Could you check a few things on this model? Use its own coordinates, in mm. Face numbers are marked on the shaded views. A direction names the side the tool comes from. Give positions to 0.01 mm unless a question says otherwise; leave off trailing zeros. Write each loop counter-clockwise with the first axis right and the second up, starting at its lowest first coordinate (ties: lowest second). Pieces come first, ordered by that corner, then holes. Notation, with made-up numbers: (-34.5, 84) - (-15.5, 84) arc R31 ccw to (-15.5, 119) - close; hole circle Ø3 at (35, 14.25). An arc over 180 degrees is marked (long way). Answer as a JSON object with one key per item and string values. Group by question number.
```python
from build123d import *

# Parameters (mm, degrees)
F1_DEPTH = 7.366
F2_T     = -1.27
F4_DEPTH = 0.762


with BuildPart() as f1:
    # F0 (on Top) → F1 (new body)
    with BuildSketch(Plane.XY):
        Polygon((14.39459, 28.100452), (3.467799, 28.100452), (-1.228805, 15.256678), (3.467799, 3.563094), (8.931195, 3.563094), (14.39459, 3.563094), (19.091195, 15.256678), align=None)
    extrude(amount=F1_DEPTH)

    # F2
    f2_openings = [f1.faces().sort_by_distance(p)[0] for p in [
        (8.931195, 28.100452, 3.683),
        (16.742892, 21.678565, 3.683),
        (16.742892, 9.409886, 3.683),
        (1.119497, 21.678565, 3.683),
        (1.119497, 9.409886, 3.683),
    ]]
    offset(amount=F2_T, openings=f2_openings)

    # F3 (on face) → F4 (join)
    with BuildSketch(Plane.XY.offset(7.366)):
        Polygon((3.955232, 13.371391), (13.296179, 13.371391), (8.625706, 21.460889), align=None)
        with BuildLine():
            ThreePointArc((7.451111, 14.032797), (7.055542, 15.560872), (8.146025, 16.702071))
            Line((8.146025, 16.702071), (8.146025, 14.032797))
            Line((8.146025, 14.032797), (7.451111, 14.032797))
        make_face(mode=Mode.SUBTRACT)
        with BuildLine():
            ThreePointArc((9.105387, 16.702071), (10.195869, 15.560872), (9.8003, 14.032797))
            Line((9.8003, 14.032797), (9.105387, 14.032797))
            Line((9.105387, 14.032797), (9.105387, 16.702071))
        make_face(mode=Mode.SUBTRACT)
        with BuildLine():
            Line((6.813301, 14.032797), (5.10082, 14.032797))
            Line((5.10082, 14.032797), (8.146025, 19.307246))
            Line((8.146025, 19.307246), (8.146025, 17.227563))
            ThreePointArc((8.146025, 17.227563), (6.659733, 15.972221), (6.813301, 14.032797))
        make_face(mode=Mode.SUBTRACT)
        with BuildLine():
            Line((9.105387, 19.307246), (12.150591, 14.032797))
            Line((12.150591, 14.032797), (10.438111, 14.032797))
            ThreePointArc((10.438111, 14.032797), (10.591678, 15.972221), (9.105387, 17.227563))
            Line((9.105387, 17.227563), (9.105387, 19.307246))
        make_face(mode=Mode.SUBTRACT)
    extrude(amount=F4_DEPTH)


solid = f1.part
```
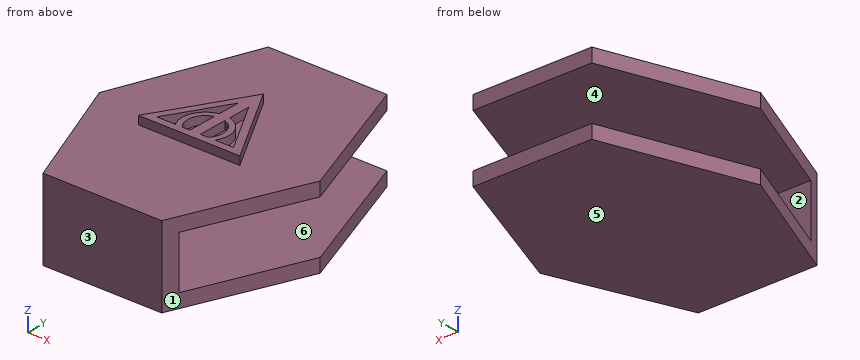
(1) I need wall thicknesses on L1, parallel to Z at x = 9.5, y = 23.5; L2, parallel to Y at x = 4.75, z = 2.25; L3, parallel to Y at x = 4.25, z = 7.75. Which ranges of each line are inside material? Lowest first, please.
(2) For the marked faces 1 and 2, which set-ups out of +Z, -Z, +X, -X, +Y, -Y let a thin tool reach every point of the face, with its end or its side?
(3) I want a section at D-D, the plane z = 2.75. Please give me the cut outline in (x, y), and give its area (3 significant figures).
(4) I want a section at B-B, the plane y = 8.5. Please give me the cut outline in (x, z).
(5) If we mould it in two halves opening along Z, with no side actions, what happens to the marked faces 3, 4, 5 and 6? For each: +Z half, -Z half, draft (parallel to the pull), parting line (faces both ways), or undercut.
(6) I want a section at C-C, the plane x = 13. Please give me the cut outline in (y, z), and give its area (3 significant figures).
(7) I want a section at A-A, the plane x = 16. Please give me the cut outline in (y, z), and give its area (3 significant figures).
(8) Will these pins go through, and if not, where does the flat tip stop? P1, Ø1, axis at x = 6.5, y = 24.5, coming from the +Z side; P2, Ø2, axis at y = 16, z = 5, coming from the -X side; P3, Ø2, axis at y = 8.5, z = 1, coming from the +X side; P4, Ø0.6, axis at y = 18, z = 7.5, coming from the -X side.
Entries:
{
 "1": {"L1": "0 to 1.27, 6.1 to 7.37", "L2": "3.56 to 4.83", "L3": "13.37 to 13.88"},
 "2": {"face 1": "+Z, -Z, +X, -Y", "face 2": "+X, -X, +Y"},
 "3": {"outline": "(2.96, 4.83) - (3.47, 3.56) - (14.39, 3.56) - (14.9, 4.83) - close", "area": "14.5 mm^2"},
 "4": {"outline": "(1.48, 0) - (16.38, 0) - (16.38, 1.27) - (1.48, 1.27) - close; (1.48, 6.1) - (16.38, 6.1) - (16.38, 7.37) - (1.48, 7.37) - close"},
 "5": {"face 3": "draft", "face 4": "undercut", "face 5": "-Z half", "face 6": "undercut"},
 "6": {"outline": "(3.56, 0) - (28.1, 0) - (28.1, 1.27) - (4.83, 1.27) - (4.83, 6.1) - (28.1, 6.1) - (28.1, 7.37) - (13.88, 7.37) - (13.88, 8.13) - (13.37, 8.13) - (13.37, 7.37) - (3.56, 7.37) - close", "area": "68.8 mm^2"},
 "7": {"outline": "(7.56, 0) - (23.71, 0) - (23.71, 1.27) - (7.56, 1.27) - close; (7.56, 6.1) - (23.71, 6.1) - (23.71, 7.37) - (7.56, 7.37) - close", "area": "41.0 mm^2"},
 "8": {"P1": "z = 7.37", "P2": "through", "P3": "x = 16.78", "P4": "x = -0.32"}
}
